Job drawing, mm, ordinate dimensions from the low corner. One solid piece. A direction names the side the tool comes from. Give positions to 0.01 mm unless a question says otherwise; leave off trailing zeros. Loops run counter-clockwise (first coordinate to the right, second up) from the corner with the lowest first, then second, coordinate; pieces in that order, holes last.
Item 1: Drop flat-ended pins along their axis: P1, Ø4, axis at x = 2.5, z = 3.5, coming from the -Y side; P2, Ø1.2, axis at x = 4.5, y = 16, coming from the +Z side (3 decimals); P3, Ø0.8, axis at x = 3.5, y = 16, coming from the -Z side; P4, Ø2, axis at x = 1.5, z = 6.5, coming from the -Y side. Give the stop position or say it passes through.
Item 2: Saw through at D-D on y = 9.25. Give the cut face in (x, z).
Item 3: Saw through at B-B on x = 3.6. Give the cut face in (y, z).
Item 4: Saw through at A-A on z = 3.6. Give the cut face in (x, y).
Item 5: Which spindle directions (+Z, -Z, +X, -X, +Y, -Y) get a long thin tool onto all of the face, cutting with end or side? Do the marked faces 4, 5 and 6. Say none if no direction does.
Item 6: Probe probe 1 along Y at (x, z) = (2.75, 3.25); probe 2 along Y at (x, z) = (5.5, 2.25); probe 3 along Z at (x, y) = (4.5, 16.25). List the from-to ranges inside material, lowest first.
Item 7: Mould opens along Z. For the marked faces 1, 2 and 3 say: released by +Z, released by -Z, zero draft, split by the parting line, or undercut.
Item 8: Saw through at C-C on y = 4.75. Give the cut face in (x, z).
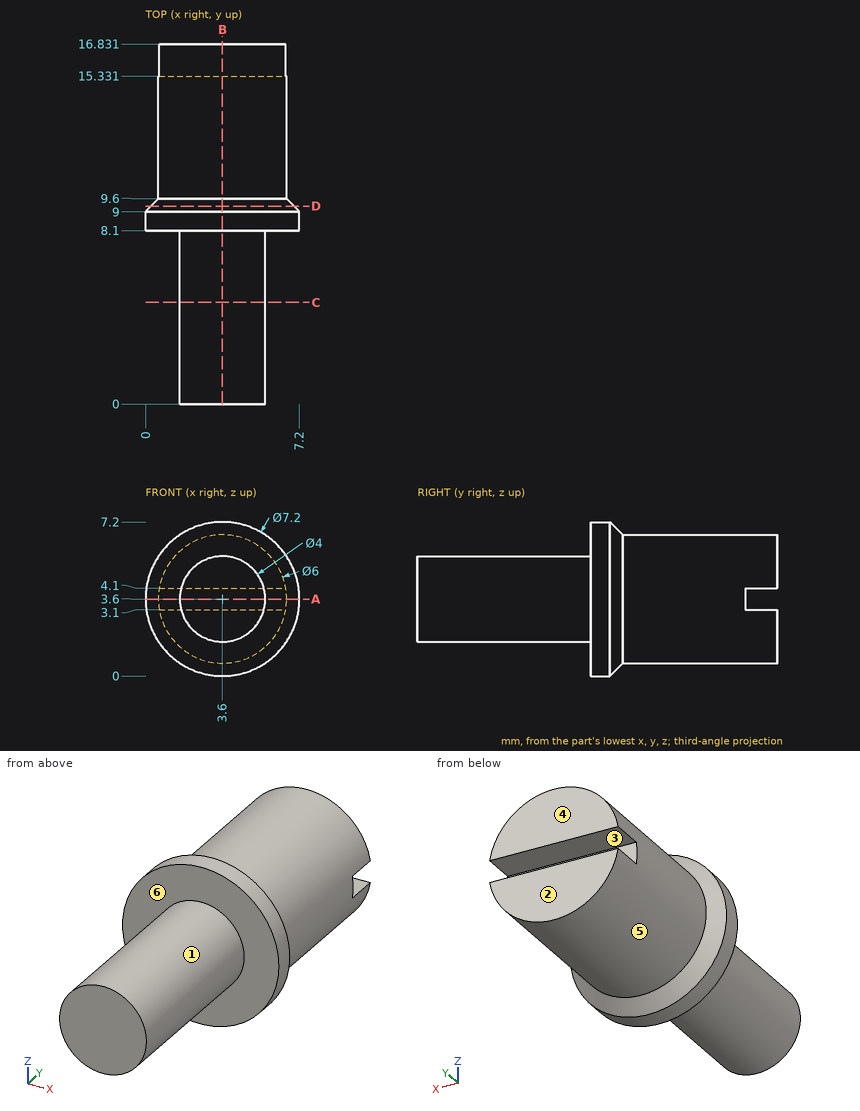
Results below:
1. P1: stops at y = 0
1. P2: stops at z = 6.585
1. P3: stops at z = 0.6
1. P4: stops at y = 8.1
2. outline: circle Ø6.7 at (3.6, 3.6)
3. outline: (0, 1.6) - (8.1, 1.6) - (8.1, 0) - (9, 0) - (9.6, 0.6) - (16.83, 0.6) - (16.83, 3.1) - (15.33, 3.1) - (15.33, 4.1) - (16.83, 4.1) - (16.83, 6.6) - (9.6, 6.6) - (9, 7.2) - (8.1, 7.2) - (8.1, 5.6) - (0, 5.6) - close
4. outline: (0, 8.1) - (1.6, 8.1) - (1.6, 0) - (5.6, 0) - (5.6, 8.1) - (7.2, 8.1) - (7.2, 9) - (6.6, 9.6) - (6.6, 15.33) - (0.6, 15.33) - (0.6, 9.6) - (0, 9) - close
5. face 4: +Z, -Z, +X, -X, +Y
5. face 5: +Y
5. face 6: -Y
6. probe 1: y = 0 to 15.33
6. probe 2: y = 8.1 to 16.83
6. probe 3: z = 0.74 to 3.1, 4.1 to 6.46
7. face 1: split by the parting line
7. face 2: zero draft
7. face 3: undercut
8. outline: circle Ø4 at (3.6, 3.6)
